from build123d import *

# Parameters (mm, degrees)
F1_DEPTH  = 120
F3_R      = 50
F4_R      = 50
F5_R      = 50
F6_R      = 50
F10_R     = 10
F11_DEPTH = 46.7291894633


with BuildPart() as f1:
    # F0 (on Front) → F1 (new body)
    with BuildSketch(Plane.XZ):
        Polygon((500, 74.5809494637), (0, 74.5809494637), (-500, 74.5809494637), (-494.533863598, 43.5809494637), (0, 43.5809494637), (494.533863598, 43.5809494637), align=None)
    extrude(amount=F1_DEPTH)

    # F2: F1 across plane


with BuildPart() as f1_1:
    add(f1.part)
    add(f1.part.mirror(Plane.XZ))

    # F3
    f3_edges = [f1_1.edges().sort_by_distance(p)[0] for p in [
        (497.266932, -120, 59.080949),
    ]]
    fillet(f3_edges, radius=F3_R)

    # F4
    f4_edges = [f1_1.edges().sort_by_distance(p)[0] for p in [
        (497.266932, 120, 59.080949),
    ]]
    fillet(f4_edges, radius=F4_R)

    # F5
    f5_edges = [f1_1.edges().sort_by_distance(p)[0] for p in [
        (-497.266932, -120, 59.080949),
    ]]
    fillet(f5_edges, radius=F5_R)

    # F6
    f6_edges = [f1_1.edges().sort_by_distance(p)[0] for p in [
        (-497.266932, 120, 59.080949),
    ]]
    fillet(f6_edges, radius=F6_R)

    # F10 (on line) → F11 (cut, through all)
    with BuildSketch(Plane(origin=(0.4902014334, 0, 2.7800704771), x_dir=(0.984807753, 0, -0.1736481777), z_dir=(0.1736481777, 0, 0.984807753))):
        with Locations((-355.8970777407, 70)):
            Circle(F10_R)
    extrude(amount=-F11_DEPTH, mode=Mode.SUBTRACT)


solid = f1_1.part
Can you work these out from the model? Positions are in its coordinate system, mm. A direction names the side the tool comes from. Round coordinates to 2 decimals unless told otherwise and drop trailing zeros. Use one line per item in the form item = value. Start each with the question number.
Q1. If I drill on probe 1 along X at (y, z) = (100, 73); probe 2 along X at (y, z) = (-94.5, 53); probe 3 along X at (y, z) = (64, 52.5), over which ranges is the centre line in solid material (lowest first)? Write a range as [from, to].
Q2. Which directions (+Z, -Z, +X, -X, +Y, -Y) give clear straight access to the entire face, cutting with the end or side of a thin tool? Please do faces 4 (the face through (-350.1, 70.1, 64.6)), 5 (the face through (482.51, 104.96, 57.49)).
Q3. We'd pull the mould along X, two halves only. Please class faces 1 (the face through (-361.83, 70.44, 55.03)), 2 (the face through (7, -2, 74.581)), 3 (the face through (-481.645, -105.742, 57.073)): +X half, -X half, draft (parallel to the pull), parting line (faces both ways), or undercut.
Q4. I'm going to push flat-ended pins straight in: P1, Ø1.5, axis at y = 9, z = 51, coming from the +X side; P2, Ø6, axis at y = -94.5, z = 57, coming from the -X side; P3, Ø4, axis at y = 18.5, z = 69.5, coming from the +X side. Where does each tip first touch, or does it pass through?
Worked out:
q1.probe_1 = [-489.57, 489.57]
q1.probe_2 = [-489.68, 489.68]
q1.probe_3 = [-496.11, -360.25], [-344.01, 496.11]
q2.face_4 = none
q2.face_5 = -Z, +X, +Y
q3.face_1 = undercut
q3.face_2 = draft
q3.face_3 = -X half
q4.P1 = 495.97
q4.P2 = -492.06
q4.P3 = 499.46
